Geometry: final body of the model. Coordinates: model frame, mm. A direction names the side the tool comes from. Round coordinates to 2 decimals unless told otherwise and drop trailing zeros. Loops run counter-clockwise (first coordinate to the right, second up) from the corner with the lowest first, then second, coordinate; pieces in that order, holes last. Notation, with made-up numbers: M 87.5,54 L 114.5,54 A32 cw 114.5,86 Z; hole C 78,49 d7. An arc over 180 degrees is marked long. Write each question's results on one line, items separated by ' | '.
```python
from build123d import *

# Parameters (mm, degrees)
SCHIZZO1_W = 2
SCHIZZO1_H = 10.457904347


with BuildPart() as part:
    # Schizzo1 → Rivoluzione1 (revolve)
    with BuildSketch(Plane.XY, mode=Mode.PRIVATE) as rivoluzione1_sk:
        Polygon((-20, 40), (-20, 0), (-14, 0), (-14, 35), (0, 35), (0, 40), align=None)
        with Locations((-19, -5.228952174)):
            Rectangle(SCHIZZO1_W, SCHIZZO1_H)
    revolve(rivoluzione1_sk.sketch.rotate(Axis((0, 0, 0), (0, 1, 0)), 270), axis=Axis((0, 0, 0), (0, 1, 0)))


solid = part.part
```
1. Draft query along Z for faces 3 (the face through (0, 40, 0)), 4 (the face through (19.524, 14.418, 4.336)), 5 (the face through (0, 35, 0)). Return one class per face: pulls with the +Z half, pulls with the -Z half, needs draft (parallel to the pull), parting line crosses it, or undercut.
Answer key:
face 3: needs draft | face 4: parting line crosses it | face 5: undercut
2. Section B-B (z = 0). Output: boundary loops of the cut face in (x, y).
Answer key:
outline: M -20,-10.46 L -18,-10.46 L -18,0 L -14,0 L -14,35 L 14,35 L 14,0 L 18,0 L 18,-10.46 L 20,-10.46 L 20,40 L -20,40 Z
3. Section D-D (y = 18). Output: boundary loops of the cut face in (x, z), then the cut area to 3 significant figures.
Answer key:
outline: C 0,0 d40; hole C 0,0 d28 | area: 641 mm²
4. Section A-A (x = 0). Output: boundary loops of the cut face in (y, z), then the cut area to 3 significant figures.
Answer key:
outline: M -10.46,-20 L 40,-20 L 40,20 L -10.46,20 L -10.46,18 L 0,18 L 0,14 L 35,14 L 35,-14 L 0,-14 L 0,-18 L -10.46,-18 Z | area: 662 mm²
5. Section C-C (y = -6). Output: boundary loops of the cut face in (x, z).
Answer key:
outline: C 0,0 d40; hole C 0,0 d36
6. Ray query, probe 1 along X at (y, z) = (-2, 0); probe 2 along X at (y, z) = (14, 0); probe 3 along Y at (x, z) = (-3, -8.5). Return the intervals inside material, ascending.
Answer key:
probe 1: x = -20 to -18, 18 to 20 | probe 2: x = -20 to -14, 14 to 20 | probe 3: y = 35 to 40
7. Pin query (flat end, axial travel): P1, Ø6, axis at y = 28, z = -7, coming from the -X side; P2, Ø5, axis at x = -6, y = -2.5, coming from the +Z side; P3, Ø22.5, axis at x = 2, z = 5.5, coming from the -Y side. Return the tip coordinate at first contact, or that it passes through.
Answer key:
P1: stops at x = -19.6 | P2: stops at z = 19.69 | P3: stops at y = 0
8. Access query for faces 1 (the face through (-3, -10.458, 18)), 2 (the face through (-5.407, -5.156, -17.169)). Directions: +Z, -Z, +X, -X, +Y, -Y. A direction counts if a zero-diameter tool reaches every point of the face in a straight line with its end or side. Return the directions, or none.
Answer key:
face 1: +Z, -Z, +X, -X, -Y | face 2: -Y
